```python
from build123d import *

# Parameters (mm, degrees)
BOSS_EXTRUDE1_DEPTH = 15
FILLET1_R           = 6
FILLET2_R           = 0.5
CUT_EXTRUDE1_DEPTH  = 74.800406503
SKETCH3_R           = 2.75
CUT_EXTRUDE2_DEPTH  = 71.582351894
SKETCH4_R           = 2.75
CUT_EXTRUDE3_DEPTH  = 74.04702868


with BuildPart() as part:
    # Sketch1 → Boss-Extrude1 (new body)
    with BuildSketch(Plane(origin=(0, 0, 0), x_dir=(1, 0, 0), z_dir=(0, 1, 0))):
        Polygon((0, 0), (-59, 0), (-59, 6), (-27.550911023, 6), (-23.724076699, 15.238795325), (-45.961940777, 37.476659403), (-41.71930009, 41.71930009), align=None)
    extrude(amount=BOSS_EXTRUDE1_DEPTH)

    # Fillet1
    fillet1_edges = [part.edges().sort_by_distance(p)[0] for p in [
        (-45.961940777, 7.5, -37.476659403),
        (-59, 7.5, -6),
    ]]
    fillet(fillet1_edges, radius=FILLET1_R - 0.0001)  # a hair under: the kernel refuses the full size

    # Fillet2
    fillet2_edges = [part.edges().sort_by_distance(p)[0] for p in [
        (0, 7.5, 0),
    ]]
    fillet(fillet2_edges, radius=FILLET2_R)

    # Sketch2 → Cut-Extrude1 (cut, through all)
    with BuildSketch(Plane(origin=(0, 15, 0), x_dir=(1, 0, 0), z_dir=(0, 1, 0))):
        Polygon((-20.185335418, 15.942694731), (-7.242640687, 3), (-25.546375109, 3), align=None)
    extrude(amount=-CUT_EXTRUDE1_DEPTH, mode=Mode.SUBTRACT)

    # Sketch3 → Cut-Extrude2 (cut, through all)
    with BuildSketch(Plane(origin=(0, 0, -6), x_dir=(-1, 0, 0), z_dir=(0, 0, -1))):
        with Locations((45, 7.5)):
            Circle(SKETCH3_R)
    extrude(amount=-CUT_EXTRUDE2_DEPTH, mode=Mode.SUBTRACT)

    # Sketch4 → Cut-Extrude3 (cut, through all)
    with BuildSketch(Plane(origin=(-4.242640687, 0, 4.242640687), x_dir=(0.7071067811865465, 0, 0.7071067811865486), z_dir=(-0.7071067811865486, 0, 0.7071067811865465))):
        with Locations((-45, 7.5)):
            Circle(SKETCH4_R)
    extrude(amount=-CUT_EXTRUDE3_DEPTH, mode=Mode.SUBTRACT)


solid = part.part
```
Here's how the part is built. I have some questions about the finished solid (model axes, mm). A direction names the side the tool comes from. Give positions to 0.01 mm unless a question says otherwise; leave off trailing zeros. Write each loop counter-clockwise with the first axis right and the second up, starting at its lowest first coordinate (ties: lowest second). Pieces come first, ordered by that corner, then holes. Notation, with made-up numbers: (-35, 83) -> (18, 83) arc R19 ccw to (18, 117) -> close; hole circle Ø7 at (48, 22.25). An arc over 180 degrees is marked (long way). Write each question's results on one line, items separated by ' | '.
Item 1: For pin 1 Ø7.5 at (x, y) = (-35, 11) entering from -Z; pin 2 Ø1 at (y, z) = (3, -22) entering from -X; pin 3 Ø4 at (y, z) = (5, -7) entering from +X; pin 4 Ø4 at (x, y) = (-47.5, 9) entering from +Z, each with a flat end and sliding along its axis, tell me the tip position at first contact or that it passes through.
Output:
pin 1: stops at z = -38.75 | pin 2: stops at x = -30.99 | pin 3: stops at x = -5 | pin 4: stops at z = 0
Item 2: Suppose I cut it at B-B on y = 9. Give the number of separate pieces and of enclosed holes in the cut face, plus the area to 3 significant figures.
Output:
separate pieces: 3 | enclosed holes: 1 | area: 492 mm^2
Item 3: Suppose I cut it at C-C on z = -4. Write out the boundary of the cut face in (x, y), plus the area to 3 significant figures.
Output:
outline: (-57.47, 0) -> (-25.13, 0) -> (-25.13, 15) -> (-57.47, 15) -> close; (-8.24, 0) -> (-4, 0) -> (-4, 15) -> (-8.24, 15) -> close; hole circle Ø5.5 at (-45, 7.5) | area: 525 mm^2
Item 4: If I drill on L1, parallel to Y at x = -45, z = -1.15; L2, parallel to Z at x = -12.5, y = 13.5; L3, parallel to X at y = 13.75, z = -4.5, over which ranges is the centre line in solid material (lowest first)?
Output:
L1: y = 0 to 4.75, 10.25 to 15 | L2: z = -12.5 to -8.26, -3 to 0 | L3: x = -56.97 to -24.93, -8.74 to -4.5
Item 5: Suppose I cut it at A-A on x = -45. Write out the boundary of the cut face in (y, z), plus the area to 3 significant figures.
Output:
outline: (0, -6) -> (4.75, -6) -> (4.75, 0) -> (0, 0) -> close; (10.25, -6) -> (15, -6) -> (15, 0) -> (10.25, 0) -> close | area: 57.0 mm^2
Item 6: On a 3-axis mill with a long thin cutter (end or side, diameter ignored), from which of +Z, -Z, +X, -X, +Y, -Y can I reach the whole of each face in a straight line? I mean faces 5 (the face through (-25.664, 7.395, -10.555)), 6 (the face through (-30, 7, 0)), 7 (the face through (-22.903, 7.605, -9.381)). Say none if no direction works.
Output:
face 5: -X, +Y, -Y | face 6: +Z, +X, -X, +Y, -Y | face 7: +Y, -Y
Item 7: We'd pull the mould along Y, two halves only. Please class faces 1 (the face through (-40, 7, -6)), 2 (the face through (-42.253, 7.621, -3.042)), 3 (the face through (-32.175, 6.447, -27.873)), 4 (the face through (-25, 0, -10)): pulls with the +Y half, pulls with the -Y half, needs draft (parallel to the pull), parting line crosses it, or undercut.
Output:
face 1: needs draft | face 2: undercut | face 3: undercut | face 4: pulls with the -Y half
